Design review of the part built by this model. Coordinates are the model's own, in mm. A direction names the side the tool comes from. Round coordinates to 2 decimals unless told otherwise and drop trailing zeros. Write each loop counter-clockwise with the first axis right and the second up, starting at its lowest first coordinate (ties: lowest second). Pieces come first, ordered by that corner, then holes.
from build123d import *

# Parameters (mm, degrees)
SKETCH2_R                        = 1.25
INTERNAL_MOUNTING_HOLES_DEPTH    = 4
ENDCAP_MOUNTING_HOLES_DEPTH      = 124.614783097
ENDCAP_MOUNTING_HOLES_DEPTH_BACK = 124.614783097
SKETCH3_R                        = 1.25


with BuildPart() as part:
    # Sketch1 → Base Boss (revolve)
    with BuildSketch(Plane(origin=(0, 0, 0), x_dir=(1, 0, 0), z_dir=(0, 1, 0))):
        Polygon((63.5, 20.32), (82.55, 20.32), (82.55, 15.24), (74.93, 15.24), (74.93, -20.32), (63.5, -20.32), align=None)
    revolve(axis=Axis((0, 0, 0), (0, 0, -1)))

    # Sketch2 → Internal Mounting Holes (cut)
    with BuildSketch(Plane.XY.offset(20.32)):
        with Locations((0, 68.58)):
            Circle(SKETCH2_R)
        with Locations((68.58, 0)):
            Circle(SKETCH2_R)
        with Locations((0, -68.58)):
            Circle(SKETCH2_R)
        with Locations((-68.58, 0)):
            Circle(SKETCH2_R)
    extrude(amount=-INTERNAL_MOUNTING_HOLES_DEPTH, mode=Mode.SUBTRACT)

    # Sketch3 → Endcap Mounting Holes (cut, two sides: drawn at the far end of the back side and taken through both)
    with BuildSketch(Plane(origin=(0, 0, -20.32), x_dir=(-1, 0, 0), z_dir=(0, 0, -1)).offset(-ENDCAP_MOUNTING_HOLES_DEPTH_BACK)):
        with Locations((0, 78.74)):
            Circle(SKETCH3_R)
        with Locations((46.282210766, 63.701998137)):
            Circle(SKETCH3_R)
        with Locations((74.886190093, 24.331998137)):
            Circle(SKETCH3_R)
        with Locations((74.886190093, -24.331998137)):
            Circle(SKETCH3_R)
        with Locations((46.282210766, -63.701998137)):
            Circle(SKETCH3_R)
        with Locations((0, -78.74)):
            Circle(SKETCH3_R)
        with Locations((-46.282210766, -63.701998137)):
            Circle(SKETCH3_R)
        with Locations((-74.886190093, -24.331998137)):
            Circle(SKETCH3_R)
        with Locations((-74.886190093, 24.331998137)):
            Circle(SKETCH3_R)
        with Locations((-46.282210766, 63.701998137)):
            Circle(SKETCH3_R)
    extrude(amount=ENDCAP_MOUNTING_HOLES_DEPTH + ENDCAP_MOUNTING_HOLES_DEPTH_BACK, mode=Mode.SUBTRACT)


solid = part.part
1) Add section B-B on z = -1. State the section outline as (x, y) points, and give its area (3 significant figures).
2) Add section A-A on y = 57. State the section outline as (x, z) points.
3) Add section C-C on y = -38. State the section outline as (x, z) points, and give its area (3 significant figures).
4) For P1, Ø1.5, axis at x = 46.28, y = -63.7, coming from the +Z side; P2, Ø3, axis at y = -10.5, z = 14.5, coming from the +X side; P3, Ø2, axis at y = 46.5, z = 6, coming from the +X side; P4, Ø2, axis at x = 46.5, z = 13, coming from the +Y side, all flat-tipped, find the tip position at first contact; note any pin that passes through.
5) For line 1 along Y through (x, z) = (1, -5); line 2 along Z through (x, y) = (69.5, -33), list the stretches that pass through material, from the lowest coordinate up.
6) The part is to be moulded in two halves that separate along X. For faces 1 (the face through (-18, -62, -20.32)), 2 (the face through (-13.77, 61.99, -0.28)), 3 (the face through (-59.462, 45.594, 2.789)), say which applies: pulls with the +X half, pulls with the -X half, needs draft (parallel to the pull), parting line crosses it, or undercut.
7) For faces 4 (the face through (73, 18, -15.24)), 5 (the face through (-17.895, 80.587, -17.744)), list the 3-axis set-ups (+Z, -Z, +X, -X, +Y, -Y) from which the entire face can be reached by the end or side of a thin tool; tool diameter is ignored.
Computed:
1. outline: circle Ø149.86 at (0, 0); hole circle Ø127 at (0, 0)
1. area: 4,970 mm2
2. outline: (-59.71, -20.32) - (-27.99, -20.32) - (-27.99, 20.32) - (-48.64, 20.32) - (-48.64, -15.24) - (-59.71, -15.24) - close; (27.99, -20.32) - (59.71, -20.32) - (59.71, -15.24) - (48.64, -15.24) - (48.64, 20.32) - (27.99, 20.32) - close
3. outline: (-73.28, -20.32) - (-50.87, -20.32) - (-50.87, 20.32) - (-64.58, 20.32) - (-64.58, -15.24) - (-73.28, -15.24) - close; (50.87, -20.32) - (73.28, -20.32) - (73.28, -15.24) - (64.58, -15.24) - (64.58, 20.32) - (50.87, 20.32) - close
3. area: 1,200 mm2
4. P1: passes through
4. P2: stops at x = 74.39
4. P3: stops at x = 59.53
4. P4: stops at y = 59.53
5. line 1: y = -74.92 to -63.49, 63.49 to 74.92
5. line 2: z = -20.32 to -15.24
6. face 1: needs draft
6. face 2: undercut
6. face 3: parting line crosses it
7. face 4: +Z
7. face 5: +Z, -Z
